Geometry check sheet. Reference: the model listing, model coordinates, mm. A direction names the side the tool comes from. Give positions to 0.01 mm unless a question says otherwise; leave off trailing zeros. Loops run counter-clockwise (first coordinate to the right, second up) from the corner with the lowest first, then second, coordinate; pieces in that order, holes last.
```python
from build123d import *

# Parameters (mm, degrees)
SKETCH1_R           = 30
BOSS_EXTRUDE1_DEPTH = 14
SKETCH2_R           = 15
BOSS_EXTRUDE2_DEPTH = 186
SKETCH3_R           = 3
CUT_EXTRUDE1_DEPTH  = 93


with BuildPart() as part:
    # Sketch1 → Boss-Extrude1 (new body)
    with BuildSketch(Plane.XY):
        Circle(SKETCH1_R)
    extrude(amount=BOSS_EXTRUDE1_DEPTH)

    # Sketch2 → Boss-Extrude2 (add)
    with BuildSketch(Plane.XY.offset(14)):
        with Locations(Location((0, 0, 0), (0, 0, 180))):
            Circle(SKETCH2_R)
    extrude(amount=BOSS_EXTRUDE2_DEPTH)

    # Sketch3 → Cut-Extrude1 (cut, symmetric)
    with BuildSketch(Plane(origin=(0, 0, 0), x_dir=(1, 0, 0), z_dir=(0, 1, 0))):
        with Locations(Location((0, -194, 0), (0, 0, 270))):
            Circle(SKETCH3_R)
    extrude(amount=CUT_EXTRUDE1_DEPTH, both=True, mode=Mode.SUBTRACT)


solid = part.part
```
1) Tool access check on faces 4 (the cylindrical face through (-29.97, 1.32, 6.9)), 5 (the cylindrical face through (-8.06, -12.65, 105.7)). Record the directions out of +Z, -Z, +X, -X, +Y, -Y that give a thin tool (end or side, any length) a straight path to the whole face; none if there is none.
2) Sectioned sample at D-D on z = 194. Enter the section's corners in (x, y), plus the area to 3 significant figures.
3) Depth check by flat-ended pin: P1, Ø1, axis at x = -21, y = 18, coming from the +Z side; P2, Ø3, axis at x = 9.5, z = 145, coming from the -Y side; P3, Ø4, axis at x = 5, z = 97.5, coming from the -Y side. Enter the tip coordinate at first touch or a pass-through.
4) Mould release check, pull along Z, two halves, no side actions. Record for faces 1 (the flat face through (0, 0, 0)), 2 (the flat face through (0, 0, 200)), 3 (the cylindrical face through (0.9, 0.21, 196.86)): +Z half, -Z half, draft (parallel to the pull), parting line (faces both ways), or undercut.
5) Sectioned sample at A-A on x = 0. Enter the section's corners in (y, z), plus the area to 3 significant figures.
6) Scan lines: line 1 along Z through (x, y) = (0, 2.5); line 2 along X through (y, z) = (1, 194); line 3 along Z through (x, y) = (21, 14). Record each from-to range of solid material in increasing order.
7) Sectioned sample at B-B on y = 0. Enter the section's corners in (x, z).
8) Sectioned sample at C-C on x = -12. Enter the section's corners in (y, z).
Determined:
1. face 4: +Z, -Z
1. face 5: +Z
2. outline: (-3, -14.7) - (-3, 14.7) arc R15 ccw to start; (3, -14.7) arc R15 ccw to (3, 14.7) - close
2. area: 528 mm2
3. P1: stops at z = 14
3. P2: stops at y = -12.69
3. P3: stops at y = -14.7
4. face 1: -Z half
4. face 2: +Z half
4. face 3: undercut
5. outline: (-30, 0) - (30, 0) - (30, 14) - (15, 14) - (15, 191) - (-15, 191) - (-15, 14) - (-30, 14) - close; (-15, 197) - (15, 197) - (15, 200) - (-15, 200) - close
5. area: 6,240 mm2
6. line 1: z = 0 to 191, 197 to 200
6. line 2: x = -14.97 to -3, 3 to 14.97
6. line 3: z = 0 to 14
7. outline: (-30, 0) - (30, 0) - (30, 14) - (15, 14) - (15, 200) - (-15, 200) - (-15, 14) - (-30, 14) - close; hole circle Ø6 at (0, 194)
8. outline: (-27.5, 0) - (27.5, 0) - (27.5, 14) - (9, 14) - (9, 200) - (-9, 200) - (-9, 14) - (-27.5, 14) - close
